The figure shows three views and two pictorial views of one solid part (mm, origin at its lowest corner). Answer the questions. A direction names the side the tool comes from. Round coordinates to 2 decimals unless told otherwise and drop trailing zeros. Order: outer loops, then holes, each group sorted by start corner. A loop starts at its lowest first (then second) coordinate and runs counter-clockwise, first axis right, second up. Notation, with made-up numbers: (82.25, -38.5) - (140.25, -38.5) arc R27 cw to (140.25, -11.5) - close; hole circle Ø2 at (72, 29.25). An arc over 180 degrees is marked (long way). Answer in a Markdown table with one row per item.
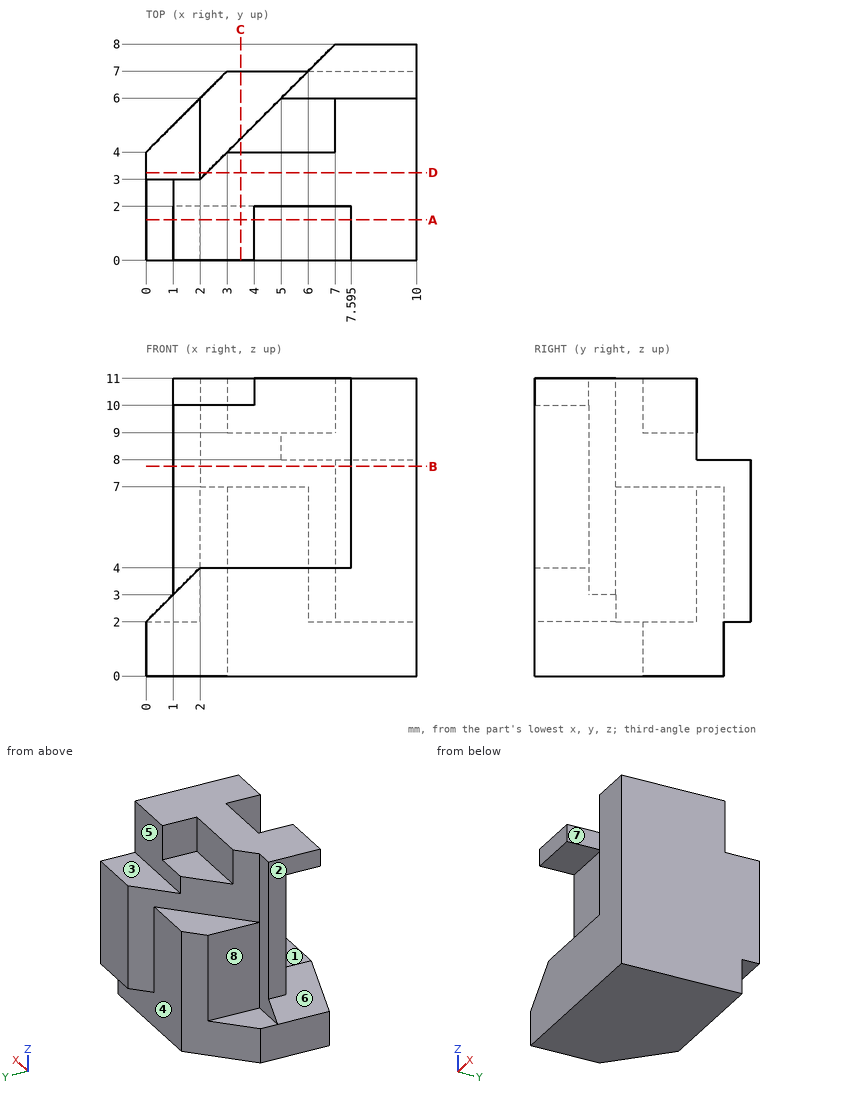
1) The mould has two halves that part along Z. Classify the marked faces 1, 2 and 3: released by +Z, released by -Z, zero draft, split by the parting line, or undercut.
Filled in:
| item | result |
|---|---|
| face 1 | undercut |
| face 2 | zero draft |
| face 3 | released by +Z |
2) Each of these flat-tipped pins is pushed along its axis until it touches: pin 1 (1.6 mm diameter, centred on x = 6, y = 0.5, fed in from +Z); pin 2 (1.5 mm diameter, centred on x = 6, z = 7, fed in from +Y); pin 3 (1 mm diameter, centred on x = 2.5, y = 5, fed in from +Z). Where does it stop, or does it pass through?
Filled in:
| item | result |
|---|---|
| pin 1 | stops at z = 4 |
| pin 2 | stops at y = 7.75 |
| pin 3 | stops at z = 7 |
3) Which of the six approach directions +Z, -Z, +X, -X, +Y, -Y give full straight-line access (tool end or side, diameter ignored) to the marked faces 4, 5, 6, 7 and 8?
Filled in:
| item | result |
|---|---|
| face 4 | -Z, -X, +Y |
| face 5 | +Z, +X, -X, +Y |
| face 6 | -X, -Y |
| face 7 | +Z, -Y |
| face 8 | +Z, -X, +Y |
4) Find section A-A, the plane y = 1.5. Give the vertices of the cut face in (x, z) (3 decimals), then the cut area to 3 significant figures.
Filled in:
| item | result |
|---|---|
| outline | (0, 0) - (10, 0) - (10, 11) - (7.595, 11) - (7.595, 4) - (2, 4) - (0, 2) - close; (1, 10) - (4, 10) - (4, 11) - (1, 11) - close |
| area | 57.8 mm^2 |
5) Find section C-C, the plane x = 3.5. Give the vertices of the cut face in (y, z), then the cut area to 3 significant figures.
Filled in:
| item | result |
|---|---|
| outline | (0, 0) - (7, 0) - (7, 7) - (4.5, 7) - (4.5, 9) - (4, 9) - (4, 11) - (0, 11) - (0, 10) - (2, 10) - (2, 4) - (0, 4) - close |
| area | 54.0 mm^2 |
6) Find section B-B, the plane z = 7.75. Give the vertices of the cut face in (x, y) (3 decimals), then the cut area to 3 significant figures.
Filled in:
| item | result |
|---|---|
| outline | (1, 2) - (7.595, 2) - (7.595, 0) - (10, 0) - (10, 8) - (7, 8) - (2, 3) - (1, 3) - close |
| area | 41.3 mm^2 |
7) Find the intervals of material crossed by probe 1 along Z at (x, y) = (5.5, 1.75); probe 2 along Y at (x, z) = (6.75, 8.5); probe 3 along Z at (x, y) = (2.5, 4), in increasing order. Write a range as from..to.
Filled in:
| item | result |
|---|---|
| probe 1 | z = 0..4 |
| probe 2 | y = 2..6 |
| probe 3 | z = 0..7 |
8) Find section D-D, the plane y = 3.25. Give the vertices of the cut face in (x, z), then the cut area to 3 significant figures.
Filled in:
| item | result |
|---|---|
| outline | (0, 0) - (10, 0) - (10, 11) - (2.25, 11) - (2.25, 7) - (2, 7) - (2, 2) - (0, 2) - close |
| area | 91.0 mm^2 |
